Here's how the part is built. I have some questions about the finished solid (model axes, mm). Coordinates: 2 decimals unless noted, no trailing zeros. Write each loop counter-clockwise with the first axis right and the second up, starting at its lowest first coordinate (ties: lowest second). Pieces come first, ordered by that corner, then holes.
```python
from build123d import *

# Parameters (mm, degrees)
BOSS_EXTRUDE1_DEPTH = 3
SKETCH4_R           = 4
CUT_EXTRUDE1_DEPTH  = 10
SKETCH6_W           = 149
SKETCH6_H           = 119
CUT_EXTRUDE2_DEPTH  = 10
SKETCH7_R           = 5
CUT_EXTRUDE3_DEPTH  = 10


with BuildPart() as part:
    # Sketch3 → Boss-Extrude1 (new body)
    with BuildSketch(Plane(origin=(0, 0, 0), x_dir=(1, 0, 0), z_dir=(0, 1, 0))):
        with BuildLine():
            Line((-150, 100), (-200, 100))
            Line((-200, 100), (-200, 167.359909647))
            ThreePointArc((-200, 167.359909647), (0, 250), (200, 167.359909647))
            Line((200, 167.359909647), (200, 100))
            Line((200, 100), (150, 100))
            Line((150, 100), (150, -100))
            Line((150, -100), (200, -100))
            Line((200, -100), (200, -167.359909647))
            ThreePointArc((200, -167.359909647), (0, -250), (-200, -167.359909647))
            Line((-200, -167.359909647), (-200, -100))
            Line((-200, -100), (-150, -100))
            Line((-150, -100), (-150, 100))
        make_face()
    extrude(amount=BOSS_EXTRUDE1_DEPTH)

    # Sketch4 → Cut-Extrude1 (cut)
    with BuildSketch(Plane(origin=(0, 3, 0), x_dir=(1, 0, 0), z_dir=(0, 1, 0))):
        with Locations(Location((-150, 167.359909647, 0), (0, 0, 270))):
            Circle(SKETCH4_R)
        with Locations(Location((150, 167.359909647, 0), (0, 0, 270))):
            Circle(SKETCH4_R)
        with Locations(Location((150, -167.359909647, 0), (0, 0, 270))):
            Circle(SKETCH4_R)
        with Locations(Location((-150, -167.359909647, 0), (0, 0, 270))):
            Circle(SKETCH4_R)
    extrude(amount=-CUT_EXTRUDE1_DEPTH, mode=Mode.SUBTRACT)

    # Sketch6 → Cut-Extrude2 (cut)
    with BuildSketch(Plane.XZ):
        Rectangle(SKETCH6_W, SKETCH6_H)
    extrude(amount=-CUT_EXTRUDE2_DEPTH, mode=Mode.SUBTRACT)

    # Sketch7 → Cut-Extrude3 (cut)
    with BuildSketch(Plane.XZ):
        with Locations(Location((-138, 26.5, 0), (0, 0, 270))):
            Circle(SKETCH7_R)
        with Locations(Location((-108, 26.5, 0), (0, 0, 270))):
            Circle(SKETCH7_R)
        with Locations(Location((108, 26.5, 0), (0, 0, 270))):
            Circle(SKETCH7_R)
        with Locations(Location((138, 26.5, 0), (0, 0, 270))):
            Circle(SKETCH7_R)
        with Locations(Location((108, -26.5, 0), (0, 0, 270))):
            Circle(SKETCH7_R)
        with Locations(Location((138, -26.5, 0), (0, 0, 270))):
            Circle(SKETCH7_R)
        with Locations(Location((-138, -26.5, 0), (0, 0, 270))):
            Circle(SKETCH7_R)
        with Locations(Location((-108, -26.5, 0), (0, 0, 270))):
            Circle(SKETCH7_R)
    extrude(amount=-CUT_EXTRUDE3_DEPTH, mode=Mode.SUBTRACT)


solid = part.part
```
1) Imagine slicing it at A-A on x = 165. Please give me the cut outline in (y, z).
Values follow:
outline: (0, -197) - (3, -197) - (3, -100) - (0, -100) - close; (0, 100) - (3, 100) - (3, 197) - (0, 197) - close
2) Will these pins go through, and if not, where does the flat tip stop? pin 1 (4 mm diameter, centred on x = -76.5, z = -109, fed in from -Y); pin 2 (1.5 mm diameter, centred on y = 1, z = 1.5, fed in from -X); pin 3 (1.5 mm diameter, centred on x = 165.5, y = 1, fed in from +Z); pin 4 (1.5 mm diameter, centred on x = -173, y = 2, fed in from +Z).
Values follow:
pin 1: stops at y = 0
pin 2: stops at x = -150
pin 3: stops at z = 197.18
pin 4: stops at z = 191.63
3) We'd pull the mould along X, two halves only. Please class faces 1 (the face through (3.108, 1.479, 249.983)), 2 (the face through (92, 3, -4)), 3 (the face through (-107.78, 1.479, 31.495)): pulls with the +X half, pulls with the -X half, needs draft (parallel to the pull), parting line crosses it, or undercut.
Values follow:
face 1: parting line crosses it
face 2: needs draft
face 3: undercut
4) I need wall thicknesses on probe 1 along X at (y, z) = (2.35, 26.5); probe 2 along X at (y, z) = (0.5, -18); probe 3 along Z at (x, y) = (-148, 0.75). Which ranges of each line are inside material? Lowest first, please.
Values follow:
probe 1: x = -150 to -143, -133 to -113, -103 to -74.5, 74.5 to 103, 113 to 133, 143 to 150
probe 2: x = -150 to -74.5, 74.5 to 150
probe 3: z = -208.27 to -170.82, -163.9 to 163.9, 170.82 to 208.27
5) Imagine slicing it at D-D on x = 10. Please give me the cut outline in (y, z).
Values follow:
outline: (0, -249.82) - (3, -249.82) - (3, -59.5) - (0, -59.5) - close; (0, 59.5) - (3, 59.5) - (3, 249.82) - (0, 249.82) - close
6) Imagine slicing it at B-B on y = 1.95. Count the separate pieces of the cut face and the enclosed holes in it, then the cut area to 3 significant figures.
Values follow:
separate pieces: 1
enclosed holes: 13
area: 141,000 mm2
7) Imagine slicing it at C-C on z = -76. Please give me the cut outline in (x, y), then the cut area to 3 significant figures.
Values follow:
outline: (-150, 0) - (150, 0) - (150, 3) - (-150, 3) - close
area: 900 mm2
